```python
from build123d import *

# Parameters (mm, degrees)
F0_R     = 17.5
F1_DEPTH = 1
F2_R     = 19
F3_DEPTH = 1
F4_R     = 3.175
F5_DEPTH = 25.4
F6_R     = 1.6383
F7_DEPTH = 25.4


with BuildPart() as f1:
    # F0 (on Front) → F1 (new body)
    with BuildSketch(Plane.XZ):
        Circle(F0_R)
    extrude(amount=F1_DEPTH)

    # F2 (on face) → F3 (join)
    with BuildSketch(Plane(origin=(0, 0, 0), x_dir=(-1, 0, 0), z_dir=(0, 1, 0))):
        Circle(F2_R)
    extrude(amount=F3_DEPTH)

    # F4 (on face) → F5 (cut)
    with BuildSketch(Plane.XZ.offset(1)):
        Circle(F4_R)
    extrude(amount=-F5_DEPTH, mode=Mode.SUBTRACT)

    # F6 (on face) → F7 (cut)
    with BuildSketch(Plane.XZ.offset(1)):
        with Locations((0, 13.3217)):
            Circle(F6_R)
        with Locations((-11.536931, -6.66085)):
            Circle(F6_R)
        with Locations((11.536931, -6.66085)):
            Circle(F6_R)
    extrude(amount=-F7_DEPTH, mode=Mode.SUBTRACT)


solid = f1.part
```
For this review, take the finished solid that the model builds, in its own axes (mm). A direction names the side the tool comes from. Round coordinates to 2 decimals unless told otherwise and drop trailing zeros. Write each loop counter-clockwise with the first axis right and the second up, starting at its lowest first coordinate (ties: lowest second). Pieces come first, ordered by that corner, then holes. Notation, with made-up numbers: (28, 28.25) - (71, 28.25) arc R20 cw to (71, 50.25) - close; hole circle Ø5 at (21, -24). An arc over 180 degrees is marked (long way). Answer as CSV lines item,"result". Start each with the question number.
(1) Add section C-C, the plane z = -6. State the section outline as (x, y) points.
(2) For pin 1 (3 mm diameter, centred on x = 11.54, z = -6.66, fed in from -Y), flat-tipped, find the tip position at first contact; note if it passes through.
(3) Add section B-B, the plane z = 0. State the section outline as (x, y) points (3 decimals).
(4) Add section A-A, the plane x = 0. State the section outline as (y, z) points (3 decimals), plus the area to 3 significant figures.
(5) Add section D-D, the plane y = 0.55. State the section outline as (x, z) points (3 decimals), plus the area to 3 significant figures.
(6) Machinability: for faces 4 (the flat face through (-6, 0, -17)), 5 (the cylindrical face through (-8.767, 0.493, -16.856)), which of the approach directions +Z, -Z, +X, -X, +Y, -Y give a long, thin tool a straight path to every point of the face, cutting with its end or side? Answer none if there is none.
(7) Mouldability with a two-part tool opening along Z and no side actions: class faces 1 (the flat face through (4, -1, 0)), 2 (the cylindrical face through (-13.887, -0.493, -10.648)), 3 (the cylindrical face through (-0.355, -0.014, 11.722)) as +Z half, -Z half, draft (parallel to the pull), parting line (faces both ways), or undercut.
(8) For line 1 (X direction, y = -0.5, z = -8); line 2 (X direction, y = -0.25, z = -6); line 3 (Z direction, x = -12.5, y = -0.05), list the stretches that pass through material, from the lowest coordinate up.
From the geometry:
1,outline,"(-18.03, 0) - (-16.44, 0) - (-16.44, -1) - (-13.04, -1) - (-13.04, 1) - (-18.03, 1) - close; (-10.04, -1) - (10.04, -1) - (10.04, 1) - (-10.04, 1) - close; (13.04, -1) - (16.44, -1) - (16.44, 0) - (18.03, 0) - (18.03, 1) - (13.04, 1) - close"
2,pin 1,"passes through"
3,outline,"(-19, 0) - (-17.5, 0) - (-17.5, -1) - (-3.175, -1) - (-3.175, 1) - (-19, 1) - close; (3.175, -1) - (17.5, -1) - (17.5, 0) - (19, 0) - (19, 1) - (3.175, 1) - close"
4,outline,"(-1, -17.5) - (0, -17.5) - (0, -19) - (1, -19) - (1, -3.175) - (-1, -3.175) - close; (-1, 3.175) - (1, 3.175) - (1, 11.683) - (-1, 11.683) - close; (-1, 14.96) - (1, 14.96) - (1, 19) - (0, 19) - (0, 17.5) - (-1, 17.5) - close"
4,area,"53.7 mm²"
5,outline,"circle Ø38 at (0, 0); hole circle Ø3.277 at (-11.537, -6.661); hole circle Ø6.35 at (0, 0); hole circle Ø3.277 at (0, 13.322); hole circle Ø3.277 at (11.537, -6.661)"
5,area,"1,080 mm²"
6,face 4,"-Y"
6,face 5,"+Y, -Y"
7,face 1,"draft"
7,face 2,"parting line"
7,face 3,"undercut"
8,line 1,"x = -15.56 to -12.48, -10.59 to 10.59, 12.48 to 15.56"
8,line 2,"x = -16.44 to -13.04, -10.04 to 10.04, 13.04 to 16.44"
8,line 3,"z = -12.25 to -7.99, -5.34 to 12.25"
